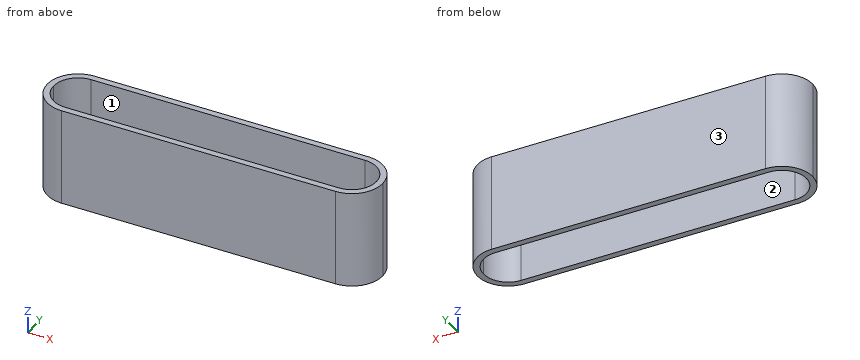
```python
from build123d import *

# Parameters (mm, degrees)
F1_DEPTH = 25


with BuildPart() as f1:
    # F0 (on Top) → F1 (new body)
    with BuildSketch(Plane.XY):
        with BuildLine():
            Line((-34.725, -7.875), (34.725, -7.875))
            ThreePointArc((34.725, -7.875), (40.293466, -5.568466), (42.6, 0))
            ThreePointArc((42.6, 0), (40.293466, 5.568466), (34.725, 7.875))
            Line((34.725, 7.875), (-34.725, 7.875))
            ThreePointArc((-34.725, 7.875), (-40.293466, 5.568466), (-42.6, 0))
            ThreePointArc((-42.6, 0), (-40.293466, -5.568466), (-34.725, -7.875))
        make_face()
        with BuildLine():
            Line((-34.725, 6.275), (34.725, 6.275))
            ThreePointArc((34.725, 6.275), (39.162095, 4.437095), (41, 0))
            ThreePointArc((41, 0), (39.162095, -4.437095), (34.725, -6.275))
            Line((34.725, -6.275), (-34.725, -6.275))
            ThreePointArc((-34.725, -6.275), (-39.162095, -4.437095), (-41, 0))
            ThreePointArc((-41, 0), (-39.162095, 4.437095), (-34.725, 6.275))
        make_face(mode=Mode.SUBTRACT)
    extrude(amount=F1_DEPTH)


solid = f1.part
```
Geometry: final body of the model. Coordinates: model frame, mm. Face numbers are marked on the shaded views. Give positions to 0.01 mm unless a question says otherwise; leave off trailing zeros. Order: outer loops, then holes, each group sorted by start corner. A loop starts at its lowest first (then second) coordinate and runs counter-clockwise, first axis right, second up. Notation, with made-up numbers: (48, 87.5) -> (98, 87.5) arc R9 ccw to (98, 95.5) -> close; hole circle Ø8 at (87.5, 21). An arc over 180 degrees is marked (long way). Write each question's results on one line, items separated by ' | '. Start each with the question number.
1) Section A-A (x = 12.5). Return loops of the section in (y, z) (3 decimals).
2) Section C-C (z = 12.75). Return loops of the section in (x, y) (3 decimals), then the cut area to 3 significant figures.
3) Draft query along X for the marked faces 1, 2 and 3. Return one class per face: pulls with the +X half, pulls with the -X half, needs draft (parallel to the pull), parting line crosses it, or undercut.
4) Line query: line 1 (Y direction, x = 29, z = 1.25) (3 decimals); line 2 (X direction, y = -1, z = 16); line 3 (Y direction, x = 39.5, z = 4.5). Output: solid intervals per line, ascending. Write a range as from..to.
5) First-contact query: pin 1 (1 mm diameter, centred on y = 0.5, z = 15.5, fed in from -X); pin 2 (1 mm diameter, centred on y = 5.5, z = 9.5, fed in from +X). Flat tips, straight axial feed; report the tip coordinate or a pass-through.
6) Section B-B (y = 0.75). Return loops of the section in (x, z), then the cut area to 3 significant figures.
Calculated:
1) outline: (-7.875, 0) -> (-6.275, 0) -> (-6.275, 25) -> (-7.875, 25) -> close; (6.275, 0) -> (7.875, 0) -> (7.875, 25) -> (6.275, 25) -> close
2) outline: (-34.725, -7.875) -> (34.725, -7.875) arc R7.875 ccw to (34.725, 7.875) -> (-34.725, 7.875) arc R7.875 ccw to start; hole (-34.725, -6.275) -> (34.725, -6.275) arc R6.275 ccw to (34.725, 6.275) -> (-34.725, 6.275) arc R6.275 ccw to start | area: 293 mm2
3) face 1: undercut | face 2: undercut | face 3: needs draft
4) line 1: -7.875..-6.275, 6.275..7.875 | line 2: -42.54..-40.92, 40.92..42.54 | line 3: -6.26..-4.07, 4.07..6.26
5) pin 1: x = -42.6 | pin 2: x = 40.81
6) outline: (-42.56, 0) -> (-40.96, 0) -> (-40.96, 25) -> (-42.56, 25) -> close; (40.96, 0) -> (42.56, 0) -> (42.56, 25) -> (40.96, 25) -> close | area: 80.5 mm2
